from build123d import *

# Parameters (mm, degrees)
SKETCH1_R      = 1.89865
MAINBODY_DEPTH = 3.175


with BuildPart() as part:
    # Sketch1 → MainBody (new body)
    with BuildSketch(Plane(origin=(0, 7.659460084, 0), x_dir=(1, 0, 0), z_dir=(0, 1, 0))):
        Polygon((-141.5163305, 104.251042847), (-124.67137867, 104.251042847), (-124.67137867, -117.799669373), (-141.5163305, -117.799669373), (-157.82954988, -6.774313263), align=None)
        with Locations(Location((-136.956490805, 82.636522264, 0), (0, 0, 270))):
            Circle(SKETCH1_R, mode=Mode.SUBTRACT)
        with Locations(Location((-142.016337919, -6.608646442, 0), (0, 0, 270))):
            Circle(SKETCH1_R, mode=Mode.SUBTRACT)
        with Locations(Location((-138.493225998, -95.927680655, 0), (0, 0, 270))):
            Circle(SKETCH1_R, mode=Mode.SUBTRACT)
    extrude(amount=-MAINBODY_DEPTH)


solid = part.part
The model under review builds one solid part; all positions refer to its coordinate system, in mm. Coordinates: 2 decimals unless noted, no trailing zeros. Loops run counter-clockwise (first coordinate to the right, second up) from the corner with the lowest first, then second, coordinate; pieces in that order, holes last. Notation, with made-up numbers: (-13.5, -21.5) -> (3.5, -21.5) arc R19 ccw to (3.5, 3.5) -> close; hole circle Ø5 at (21.25, 26). An arc over 180 degrees is marked (long way). Use a Markdown table: item, result. Add a question column.
1. Add section A-A on y = 5.05. Write out the cut boundary in (x, z), plus the area to 3 significant figures.
2. Add section C-C on x = -153.5. Write out the cut boundary in (y, z), plus the area to 3 significant figures.
3. Draft analysis for pull direction Z (two halves, no side actions). For faces 1 (the face through (-137, 4.484, 5)), 2 (the face through (-149.787, 6.094, -47.961)), 3 (the face through (-135.673, 6.094, -84.036)), 4 (the face through (-149.56, 6.09, 63.06)), state which applies: pulls with the +Z half, pulls with the -Z half, needs draft (parallel to the pull), parting line crosses it, or undercut.
4. Add section B-B on z = -78.5. Write out the cut boundary in (x, y).
5. To check wall thickness, follow line 1 (Z direction, x = -138.5, y = 5.15); line 2 (Z direction, x = -141, y = 5); line 3 (Z direction, x = -140.5, y = 6.4). State the ranges of each line that lie inside material, in increasing order.
6. Clearance check with a flat-ended pin moving along its axis: pin 1 Ø2.5 at (x, z) = (-138.49, 95.93) entering from +Y (3 decimals). State where the tip first meets the part, or that it passes through.
Returned:
| question | item | result |
|---|---|---|
| 1 | outline | (-157.83, 6.77) -> (-141.52, -104.25) -> (-124.67, -104.25) -> (-124.67, 117.8) -> (-141.52, 117.8) -> close; hole circle Ø3.8 at (-142.02, 6.61); hole circle Ø3.8 at (-138.49, 95.93); hole circle Ø3.8 at (-136.96, -82.64) |
| 1 | area | 5,520 mm² |
| 2 | outline | (4.48, -22.69) -> (7.66, -22.69) -> (7.66, 36.24) -> (4.48, 36.24) -> close |
| 2 | area | 187 mm² |
| 3 | face 1 | needs draft |
| 3 | face 2 | pulls with the -Z half |
| 3 | face 3 | undercut |
| 3 | face 4 | pulls with the +Z half |
| 4 | outline | (-145.3, 4.48) -> (-124.67, 4.48) -> (-124.67, 7.66) -> (-145.3, 7.66) -> close |
| 5 | line 1 | z = -104.25 to -83.74, -81.53 to 94.03, 97.83 to 117.8 |
| 5 | line 2 | z = -104.25 to 5, 8.21 to 117.8 |
| 5 | line 3 | z = -104.25 to 5.47, 7.75 to 117.8 |
| 6 | pin 1 | passes through |
